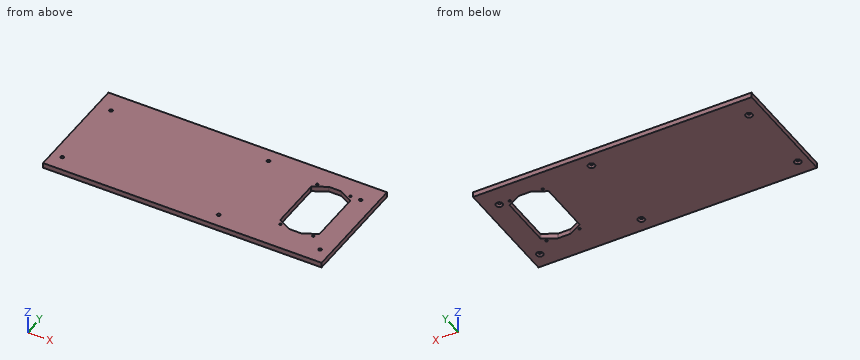
```python
from build123d import *

# Parameters (mm, degrees)
SKETCH1_W                             = 270
SKETCH1_H                             = 110
SHEET_DEPTH                           = 2.5
SKETCH4_R                             = 1.1
CUT_EXTRUDE1_DEPTH                    = 6
FILLET1_R                             = 1
F_3_2_3_2_MOUNTHOLES_D                = 3.2
F_3_2_3_2_MOUNTHOLES_CSINK_D          = 6.5
F_3_2_3_2_MOUNTHOLES_CSINK_ANGLE      = 90
F_3_2_3_2_MIDDLEPARTHOLES_D           = 3.2
F_3_2_3_2_MIDDLEPARTHOLES_CSINK_D     = 6.5
F_3_2_3_2_MIDDLEPARTHOLES_CSINK_ANGLE = 90


with BuildPart() as part:
    # Sketch1 → Sheet (new body, symmetric)
    with BuildSketch(Plane.XY):
        Rectangle(SKETCH1_W, SKETCH1_H)
    extrude(amount=SHEET_DEPTH, both=True)

    # Sketch4 → Cut-Extrude1 (cut, through all)
    with BuildSketch(Plane(origin=(0, 0, -2.5), x_dir=(-1, 0, 0), z_dir=(0, 0, -1))):
        with Locations((-79, 35)):
            Circle(SKETCH4_R)
        with Locations((-111, 35)):
            Circle(SKETCH4_R)
        with Locations((-111, -27)):
            Circle(SKETCH4_R)
        with Locations((-79, -27)):
            Circle(SKETCH4_R)
        Polygon((-101, 37), (-114, 30), (-114, -22), (-101, -29), (-89, -29), (-76, -22), (-76, 30), (-89, 37), align=None)
    extrude(amount=-CUT_EXTRUDE1_DEPTH, mode=Mode.SUBTRACT)

    # Fillet1
    fillet1_edges = [part.edges().sort_by_distance(p)[0] for p in [
        (89, 37, 0),
        (76, 30, 0),
        (76, -22, 0),
        (89, -29, 0),
        (101, -29, 0),
        (114, -22, 0),
        (114, 30, 0),
        (101, 37, 0),
    ]]
    fillet(fillet1_edges, radius=FILLET1_R)

    # Ø3.2 (3.2) MountHoles (through all)
    with Locations(Plane(origin=(0, 0, -2.5), x_dir=(-1, 0, 0), z_dir=(0, 0, -1))):
        with Locations((-121, 35), (-125, -40), (125, -40), (121, 35)):
            CounterSinkHole(F_3_2_3_2_MOUNTHOLES_D / 2, F_3_2_3_2_MOUNTHOLES_CSINK_D / 2, counter_sink_angle=F_3_2_3_2_MOUNTHOLES_CSINK_ANGLE)

    # Ø3.2 (3.2) MiddlePartHoles (through all)
    with Locations(Plane(origin=(0, 0, -2.5), x_dir=(-1, 0, 0), z_dir=(0, 0, -1))):
        with Locations((-27.7, 42), (-27.7, -42)):
            CounterSinkHole(F_3_2_3_2_MIDDLEPARTHOLES_D / 2, F_3_2_3_2_MIDDLEPARTHOLES_CSINK_D / 2, counter_sink_angle=F_3_2_3_2_MIDDLEPARTHOLES_CSINK_ANGLE)


solid = part.part
```
Can you work these out from the model? Positions are in its coordinate system, mm. Give positions to 0.01 mm unless a question says otherwise; leave off trailing zeros. Loops run counter-clockwise (first coordinate to the right, second up) from the corner with the lowest first, then second, coordinate; pieces in that order, holes last. Notation, with made-up numbers: M 74,10 L 80,10 A9 ccw 80,16 Z; hole C -34,71.5 d11. An arc over 180 degrees is marked long. Use CSV: the item, a comma, the result in double quotes. Start each with the question number.
1. Imagine slicing it at B-B, the plane z = 0.45. Count the separate pieces of the cut face and the enclosed holes in it, plus the area to 3 significant figures.
2. If I drill on L1, parallel to X at y = -40, z = 1.5; L2, parallel to X at y = 15.5, z = 0.8; L3, parallel to X at y = 42, z = 1.3, over which ranges is the centre line in solid material (lowest first)?
3. For P1, Ø5, axis at x = 121, y = 35, coming from the -Z side; P2, Ø3.5, axis at x = 27.7, y = -42, coming from the -Z side, each with a flat end and sliding along its axis, tell me the tip position at first contact or that it passes through.
4. Imagine slicing it at A-A, the plane y = -6. Write out the boundary of the cut face in (x, z).
Response values:
1,separate pieces,"1"
1,enclosed holes,"11"
1,area,"27,300 mm^2"
2,L1,"-135 to -126.6, -123.4 to 123.4, 126.6 to 135"
2,L2,"-135 to 76, 114 to 135"
2,L3,"-135 to 26.1, 29.3 to 135"
3,P1,"z = -1.75"
3,P2,"z = -1"
4,outline,"M -135,-2.5 L 76,-2.5 L 76,2.5 L -135,2.5 Z; M 114,-2.5 L 135,-2.5 L 135,2.5 L 114,2.5 Z"
